For this review, take the finished solid that the model builds, in its own axes (mm). A direction names the side the tool comes from. Coordinates: 2 decimals unless noted, no trailing zeros. Order: outer loops, then holes, each group sorted by start corner. A loop starts at its lowest first (then second) coordinate and runs counter-clockwise, first axis right, second up.
from build123d import *

# Parameters (mm, degrees)
EXTRU_MINCE1_DEPTH      = 24
ESQUISSE2_R             = 2.25
ENL_V_MAT_EXTRU_1_DEPTH = 20


with BuildPart() as part:
    # Esquisse1 → Extru.-Mince1 (new body)
    with BuildSketch(Plane.XY):
        Polygon((-2.7, -35.65), (-2.7, -20.65), (-29.7, -20.65), (-29.7, 20.65), (29.7, 20.65), (29.7, -20.65), (2.7, -20.65), (2.7, -35.65), (5.7, -35.65), (5.7, -23.65), (32.7, -23.65), (32.7, 23.65), (-32.7, 23.65), (-32.7, -23.65), (-5.7, -23.65), (-5.7, -35.65), align=None)
    extrude(amount=EXTRU_MINCE1_DEPTH)

    # Esquisse2 → Enlèv. mat.-Extru.1 (cut)
    with BuildSketch(Plane.ZY.offset(5.7)):
        with Locations(Location((12, -30.65, 0), (0, 0, 270))):
            Circle(ESQUISSE2_R)
        Polygon((0, -23.65), (7, -35.65), (0, -35.65), align=None)
        Polygon((17, -35.65), (24, -35.65), (24, -23.65), align=None)
    extrude(amount=-ENL_V_MAT_EXTRU_1_DEPTH, mode=Mode.SUBTRACT)


solid = part.part
1. To check wall thickness, follow L1, parallel to Y at x = -4, z = 9.5; L2, parallel to Y at x = 16, z = 4.5; L3, parallel to X at y = -3, z = 21.75. State the ranges of each line that lie inside material, in increasing order.
Answer below:
L1: y = -35.65 to -20.65, 20.65 to 23.65
L2: y = -23.65 to -20.65, 20.65 to 23.65
L3: x = -32.7 to -29.7, 29.7 to 32.7
2. Take a section at A-A, the plane x = 16. Give the boundary of the cut face in (y, z).
Answer below:
outline: (-23.65, 0) - (-20.65, 0) - (-20.65, 24) - (-23.65, 24) - close; (20.65, 0) - (23.65, 0) - (23.65, 24) - (20.65, 24) - close
3. Take a section at C-C, the plane z = 12. Give the boundary of the cut face in (x, y), plus the area to 3 significant figures.
Answer below:
outline: (-32.7, -23.65) - (-5.7, -23.65) - (-5.7, -28.4) - (-2.7, -28.4) - (-2.7, -20.65) - (-29.7, -20.65) - (-29.7, 20.65) - (29.7, 20.65) - (29.7, -20.65) - (2.7, -20.65) - (2.7, -28.4) - (5.7, -28.4) - (5.7, -23.65) - (32.7, -23.65) - (32.7, 23.65) - (-32.7, 23.65) - close; (-5.7, -35.65) - (-2.7, -35.65) - (-2.7, -32.9) - (-5.7, -32.9) - close; (2.7, -35.65) - (5.7, -35.65) - (5.7, -32.9) - (2.7, -32.9) - close
area: 669 mm2
4. Take a section at D-D, the plane z = 8. Give the boundary of the cut face in (x, y).
Answer below:
outline: (-32.7, -23.65) - (-5.7, -23.65) - (-5.7, -35.65) - (-2.7, -35.65) - (-2.7, -20.65) - (-29.7, -20.65) - (-29.7, 20.65) - (29.7, 20.65) - (29.7, -20.65) - (2.7, -20.65) - (2.7, -35.65) - (5.7, -35.65) - (5.7, -23.65) - (32.7, -23.65) - (32.7, 23.65) - (-32.7, 23.65) - close
5. The part is to be moulded in two halves that separate along X. For faces 5 (the face through (5.7, -28, 12)), 6 (the face through (4, -35.65, 12)), 7 (the face through (0, 20.65, 12)), say which applies: +X half, -X half, draft (parallel to the pull), parting line (faces both ways), or undercut.
Answer below:
face 5: +X half
face 6: draft
face 7: undercut
6. Take a section at B-B, the plane y = 16.5. Give the boundary of the cut face in (x, z).
Answer below:
outline: (-32.7, 0) - (-29.7, 0) - (-29.7, 24) - (-32.7, 24) - close; (29.7, 0) - (32.7, 0) - (32.7, 24) - (29.7, 24) - close
7. Machinability: for faces 1 (the face through (0, 23.65, 12)), 2 (the face through (16, -20.65, 12)), 3 (the face through (-5.7, -28, 12)), 4 (the face through (-2.7, -27, 12)), which of the approach directions +Z, -Z, +X, -X, +Y, -Y give a long, thin tool a straight path to every point of the face, cutting with its end or side? Answer none if there is none.
Answer below:
face 1: +Z, -Z, +X, -X, +Y
face 2: +Z, -Z
face 3: +Z, -Z, -X, -Y
face 4: +Z, -Z, -Y
8. Clearance check with flat-ended pins moving along their axes: pin 1 Ø6 at (y, z) = (-30.65, 12) entering from -X; pin 2 Ø3 at (x, z) = (-9, 19.5) entering from -Y; pin 3 Ø6 at (y, z) = (-30.65, 12) entering from +X. State where each tip first meets the part, or that it passes through.
Answer below:
pin 1: stops at x = -5.7
pin 2: stops at y = -23.65
pin 3: stops at x = 5.7
